Read the model definition and answer for the solid it produces. Units are mm, in the model's axes. Round coordinates to 2 decimals unless told otherwise and drop trailing zeros. Order: outer loops, then holes, each group sorted by start corner. A loop starts at its lowest first (then second) coordinate and runs counter-clockwise, first axis right, second up. Notation, with made-up numbers: M 62.25,-22 L 66.25,-22 A18 cw 66.25,6 Z; hole C 85.25,23 d5. An arc over 180 degrees is marked long. Use one line per item in the form item = value. Start each with the question number.
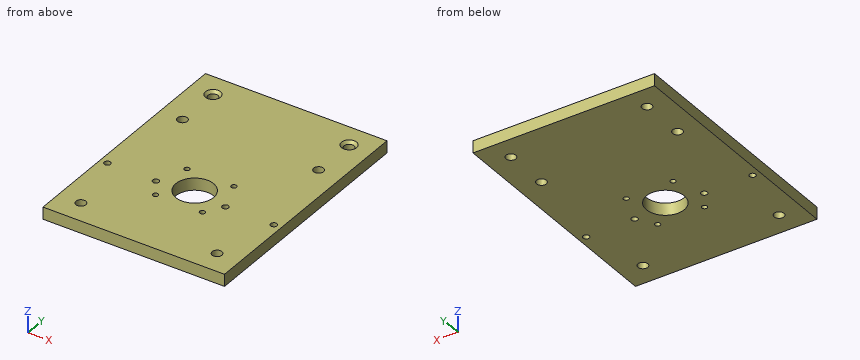
Autodesk Inventor part; units mm, degrees
ref_plane "YZ Plane" through (0, 0, 0) normal (1, 0, 0) x (0, 1, 0)
ref_plane "XZ Plane" through (0, 0, 0) normal (0, 1, 0) x (-1, 0, 0)
ref_plane "XY Plane" through (0, 0, 0) normal (0, 0, 1) x (1, 0, 0)
sketch "Sketch1" plane through (0, 0, 0) normal (0, 0, 1) x (1, 0, 0)
  line L0 (0, 0) -> (120, 0)
  line L1 (120, 0) -> (120, 160)
  line L2 (120, 160) -> (0, 160)
  line L3 (0, 160) -> (0, 0)
  dimension "width" = 120
  dimension "d1" = 160
extrude "Extrusion1" add sketch "Sketch1" along normal blind 8
hole "Hole1" at (15, 15, 8) direction (0, 0, -1) diameter 6.5 end through all
pattern_linear "Rectangular Pattern1" count 2 spacing 90 along (1, 0, 0) count 2 spacing 100 along (0, 1, 0) of "Hole1"
hole "Hole2" at (15, 145, 8) direction (0, 0, -1) diameter 6.5 end through all countersink diameter 10 countersink angle 90
pattern_linear "Rectangular Pattern2" count 2 spacing 90 along (1, 0, 0) of "Hole2"
hole "Hole3" at (60, 60, 8) direction (0, 0, -1) diameter 25 end through all
hole "Hole4" at (44.5, 75.5, 8) direction (0, 0, -1) diameter 3.5 end through all
pattern_linear "Rectangular Pattern3" count 2 spacing 31 along (0, -1, 0) count 2 spacing 31 along (1, 0, 0) of "Hole4"
hole "Hole5" at (5, 56, 8) direction (0, 0, -1) diameter 4.134 end through all
hole "Hole6" at (115, 56, 8) direction (0, 0, -1) diameter 4.134 end through all
pattern_linear "Rectangular Pattern4" count 2 spacing 32 along (1, 0, 0) of "Hole5"
pattern_linear "Rectangular Pattern5" count 2 spacing 32 along (-1, 0, 0) of "Hole6"
properties part number "motor plate support"
Item 1: Section A-A (x = 83) is taken. Write down the section's boundary in (y, z).
Item 2: Section B-B (y = 75.5) is taken. Write down the section's boundary in (x, z).
Item 3: Section C-C (x = 15) is taken. Write down the section's boundary in (y, z).
Item 4: Given P1, Ø4, axis at x = 15, y = 115, coming from the -Z side, flat-ended and moving along its own axis, determine where the tip first touches the part or whether it passes through.
Item 5: Section D-D (z = 1.5) is taken. Give the number of separate pieces and of enclosed holes in the cut face, and give its area (3 significant figures).
Item 6: Find the intervals of material crossed by L1, parallel to Y at x = 105, z = 5.5; L2, parallel to X at y = 44.5, z = 7.25; L3, parallel to X at y = 15, z = 6.5, in increasing order. Write a range as [from, to].
The answers:
q1.outline = M 0,0 L 53.93,0 L 53.93,8 L 0,8 Z; M 58.07,0 L 160,0 L 160,8 L 58.07,8 Z
q2.outline = M 0,0 L 42.75,0 L 42.75,8 L 0,8 Z; M 46.25,0 L 73.75,0 L 73.75,8 L 46.25,8 Z; M 77.25,0 L 120,0 L 120,8 L 77.25,8 Z
q3.outline = M 0,0 L 11.75,0 L 11.75,8 L 0,8 Z; M 18.25,0 L 111.75,0 L 111.75,8 L 18.25,8 Z; M 118.25,0 L 141.75,0 L 141.75,6.25 L 140,8 L 118.25,8 Z; M 148.25,0 L 160,0 L 160,8 L 150,8 L 148.25,6.25 Z
q4.P1 = through
q5.separate_pieces = 1
q5.enclosed_holes = 15
q5.area = 18,400 mm²
q6.L1 = [0, 11.75], [18.25, 111.75], [118.25, 141.75], [148.25, 160]
q6.L2 = [0, 42.75], [46.25, 73.75], [77.25, 120]
q6.L3 = [0, 11.75], [18.25, 101.75], [108.25, 120]
